from build123d import *

# Parameters (mm, degrees)
PAD004_DEPTH    = 8.2
SKETCH014_W     = 28.5
SKETCH014_H     = 6.2
PAD005_DEPTH    = 1.8
SKETCH015_R     = 2.9
POCKET004_DEPTH = 0.6
SKETCH016_W     = 2.05
SKETCH016_H     = 6.2
POCKET005_DEPTH = 1.8
SKETCH018_R     = 1.05
POCKET007_DEPTH = 6


with BuildPart() as part:
    # Sketch013 → Pad004 (new body)
    with BuildSketch(Plane.XY):
        with BuildLine():
            Line((0, 0), (28.5, 0))
            Line((28.5, 0), (28.5, 22.75))
            Line((28.5, 22.75), (14, 22.75))
            Line((14, 22.75), (14, 22.5))
            ThreePointArc((11, 19.5), (13.12132, 20.37868), (14, 22.5))
            Line((11, 19.5), (0, 19.5))
            Line((0, 19.5), (0, 0))
        make_face()
    extrude(amount=PAD004_DEPTH)

    # Sketch014 (on Face9 of Pad004) → Pad005 (join)
    with BuildSketch(Plane.XY.offset(8.2)):
        with Locations((14.25, 9.75)):
            Rectangle(SKETCH014_W, SKETCH014_H)
    extrude(amount=PAD005_DEPTH)

    # Sketch015 (on Face11 of Pad005) → Pocket004 (cut)
    with BuildSketch(Plane.XY.offset(10)):
        with Locations((8.735056, 9.75)):
            Circle(SKETCH015_R)
    extrude(amount=-POCKET004_DEPTH, mode=Mode.SUBTRACT)

    # Sketch016 (on Face10 of Pocket004) → Pocket005 (cut)
    with BuildSketch(Plane.XY.offset(10)):
        with Locations((15.5, 9.75)):
            Rectangle(SKETCH016_W, SKETCH016_H)
        Polygon((21.525, 12.85), (21.525, 6.65), (19.475, 6.65), (19.475, 12.85), (20.5, 12.85), align=None)
        with Locations((25.5, 9.75)):
            Rectangle(SKETCH016_W, SKETCH016_H)
    extrude(amount=-POCKET005_DEPTH, mode=Mode.SUBTRACT)

    # Sketch018 (on Face19 of Clone001) → Pocket007 (cut)
    with BuildSketch(Plane.XY.offset(8.2)):
        with BuildLine():
            Line((14, 22.75), (26.9, 22.75))
            Line((26.9, 22.75), (26.9, 16.25))
            Line((26.355184, 16.25), (26.9, 16.25))
            ThreePointArc((21.044816, 16.25), (23.7, 14.75), (26.355184, 16.25))
            Line((20.45, 16.25), (21.044816, 16.25))
            Line((19.855184, 16.25), (20.45, 16.25))
            ThreePointArc((14.544816, 16.25), (17.2, 14.75), (19.855184, 16.25))
            Line((14, 16.25), (14.544816, 16.25))
            Line((14, 16.25), (14, 22.75))
        make_face()
        with Locations((17.2, 17.85)):
            Circle(SKETCH018_R, mode=Mode.SUBTRACT)
        with Locations((23.7, 17.85)):
            Circle(SKETCH018_R, mode=Mode.SUBTRACT)
    extrude(amount=-POCKET007_DEPTH, mode=Mode.SUBTRACT)


solid = part.part
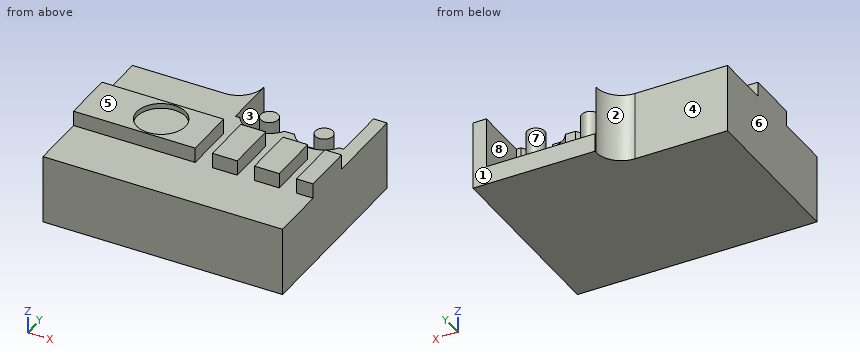
Input: part model. Units: mm. Frame: model coordinates. Face numbers are marked on the shaded views. A direction names the side the tool comes from. Coordinates: 2 decimals unless noted, no trailing zeros. Order: outer loops, then holes, each group sorted by start corner. A loop starts at its lowest first (then second) coordinate and runs counter-clockwise, first axis right, second up. Notation, with made-up numbers: M 5,61 L 55,61 A19 cw 55,72 Z; hole C 89,34.25 d3. An arc over 180 degrees is marked long. One line per question, with ' | ' between items.
Item 1: Section A-A (z = 4.25). Output: boundary loops of the cut face in (x, y), then the cut area to 3 significant figures.
Geometry results:
outline: M 0,0 L 28.5,0 L 28.5,22.75 L 26.9,22.75 L 26.9,16.25 L 26.36,16.25 A3.1 cw 21.04,16.25 L 19.86,16.25 A3.1 cw 14.54,16.25 L 14,16.25 L 14,22.5 A3 cw 11,19.5 L 0,19.5 Z; C 17.2,17.85 d2.1; C 23.7,17.85 d2.1 | area: 517 mm^2
Item 2: Draft query along X for the marked faces 1, 2 and 3. Return one class per face: released by +X, released by -X, zero draft, split by the parting line, or undercut.
Geometry results:
face 1: zero draft | face 2: released by -X | face 3: undercut
Item 3: Section C-C (y = 17.85). Output: boundary loops of the cut face in (x, z).
Geometry results:
outline: M 0,0 L 28.5,0 L 28.5,8.2 L 26.9,8.2 L 26.9,2.2 L 24.75,2.2 L 24.75,8.2 L 22.65,8.2 L 22.65,2.2 L 18.25,2.2 L 18.25,8.2 L 16.15,8.2 L 16.15,2.2 L 14,2.2 L 14,8.2 L 0,8.2 Z
Item 4: Reachability of the marked faces 4, 5, 6, 7 and 8 from +Z, -Z, +X, -X, +Y, -Y: full face, straight path, thin tool, end or side. Return the list, or none.
Geometry results:
face 4: +Z, -Z, -X, +Y | face 5: +Z, +X, -X, +Y, -Y | face 6: +Z, -Z, -X, +Y, -Y | face 7: +Z | face 8: +Z, +Y
Item 5: Section B-B (z = 9). Output: boundary loops of the cut face in (x, y) (3 decimals), then the cut area to 3 significant figures.
Geometry results:
outline: M 0,6.65 L 14.475,6.65 L 14.475,12.85 L 0,12.85 Z; M 16.525,6.65 L 19.475,6.65 L 19.475,12.85 L 16.525,12.85 Z; M 21.525,6.65 L 24.475,6.65 L 24.475,12.85 L 21.525,12.85 Z; M 26.525,6.65 L 28.5,6.65 L 28.5,12.85 L 26.525,12.85 Z | area: 139 mm^2
Item 6: Section D-D (x = 23.7). Output: boundary loops of the cut face in (y, z).
Geometry results:
outline: M 0,0 L 22.75,0 L 22.75,2.2 L 18.9,2.2 L 18.9,8.2 L 16.8,8.2 L 16.8,2.2 L 14.75,2.2 L 14.75,8.2 L 12.85,8.2 L 12.85,10 L 6.65,10 L 6.65,8.2 L 0,8.2 Z
Item 7: Ray query, line 1 along X through (y, z) = (18.75, 6.5); line 2 along X through (y, z) = (19.25, 8); line 3 along Y through (x, z) = (13.25, 9.75). Return the intervals inside material, ascending.
Geometry results:
line 1: x = 0 to 14, 16.66 to 17.74, 23.16 to 24.24, 26.9 to 28.5 | line 2: x = 0 to 14, 26.9 to 28.5 | line 3: y = 6.65 to 12.85
Item 8: Pin query (flat end, axial travel): pin 1 (8 mm diameter, centred on x = 16.5, y = 2.5, fed in from +Z); pin 2 (3 mm diameter, centred on x = 5.5, z = 1.5, fed in from +Y); pin 3 (2 mm diameter, centred on x = 23, z = 9.5, fed in from +Y). Return the tip coordinate at first contact, or that it passes through.
Geometry results:
pin 1: stops at z = 8.2 | pin 2: stops at y = 19.5 | pin 3: stops at y = 12.85
